from build123d import *

# Parameters (mm, degrees)
SKETCH1_W          = 73.81875
SKETCH1_H          = 114.3
BASE_FLANGE1_DEPTH = 1.5875
EDGE_FLANGE1_DEPTH = 114.3
SKETCH11_R         = 2.45745
CUT_EXTRUDE1_DEPTH = 155.799566224
SKETCH12_R         = 2.45745
CUT_EXTRUDE2_DEPTH = 156.949151494
FILLET1_R          = 2.54


# Sheet-metal steps are written as plain solids
with BuildPart() as part:
    # Sketch1 → Base-Flange1 (new body)
    with BuildSketch(Plane.XY):
        with Locations((36.909375, 57.15)):
            Rectangle(SKETCH1_W, SKETCH1_H)
    extrude(amount=-BASE_FLANGE1_DEPTH)

    # Edge-Flange1 section (across the edge) → Edge-Flange1 (add)
    with BuildSketch(Plane(origin=(-0.79375, 0, -1.5875), x_dir=(1, 0, 0), z_dir=(0, 1, 0))):
        with BuildLine():
            Line((-1.5875, 0.79375), (-1.5875, 72.23125))
            Line((-1.5875, 72.23125), (0, 72.23125))
            Line((0, 72.23125), (0, 0.79375))
            ThreePointArc((0, 0.79375), (0.232483992, 0.232483992), (0.79375, 0))
            Line((0.79375, 0), (0.79375, -1.5875))
            ThreePointArc((0.79375, -1.5875), (-0.890048023, -0.890048023), (-1.5875, 0.79375))
        make_face()
    extrude(amount=EDGE_FLANGE1_DEPTH)

    # Sketch11 → Cut-Extrude1 (cut, through all)
    with BuildSketch(Plane.XY):
        with Locations((30.48, 12.7)):
            Circle(SKETCH11_R)
        with Locations((30.48, 33.02)):
            Circle(SKETCH11_R)
        with Locations((30.48, 53.34)):
            Circle(SKETCH11_R)
        with Locations((30.48, 73.66)):
            Circle(SKETCH11_R)
        with Locations((30.48, 93.98)):
            Circle(SKETCH11_R)
        with Locations((61.11875, 101.6)):
            Circle(SKETCH11_R)
        with Locations((61.11875, 81.28)):
            Circle(SKETCH11_R)
        with Locations((61.11875, 60.96)):
            Circle(SKETCH11_R)
        with Locations((61.11875, 40.64)):
            Circle(SKETCH11_R)
        with Locations((61.11875, 20.32)):
            Circle(SKETCH11_R)
        with BuildLine():
            Line((46.67885, 88.10625), (43.50385, 88.10625))
            ThreePointArc((43.50385, 88.10625), (36.3601, 95.25), (43.50385, 102.39375))
            Line((43.50385, 102.39375), (46.67885, 102.39375))
            ThreePointArc((46.67885, 102.39375), (53.8226, 95.25), (46.67885, 88.10625))
        make_face()
        with BuildLine():
            Line((46.67885, 11.90625), (43.50385, 11.90625))
            ThreePointArc((43.50385, 11.90625), (36.3601, 19.05), (43.50385, 26.19375))
            Line((43.50385, 26.19375), (46.67885, 26.19375))
            ThreePointArc((46.67885, 26.19375), (53.8226, 19.05), (46.67885, 11.90625))
        make_face()
        with BuildLine():
            Line((43.383061388, 65.139055024), (40.208061388, 63.488055024))
            ThreePointArc((40.208061388, 63.488055024), (36.3601, 57.15), (40.208061388, 50.811944976))
            Line((40.208061388, 50.811944976), (43.383061388, 49.160944976))
            ThreePointArc((43.383061388, 49.160944976), (50.386199064, 49.392550378), (53.8226, 55.499))
            Line((53.8226, 55.499), (53.8226, 58.801))
            ThreePointArc((53.8226, 58.801), (50.386199064, 64.907449622), (43.383061388, 65.139055024))
        make_face()
    extrude(amount=-CUT_EXTRUDE1_DEPTH, mode=Mode.SUBTRACT)

    # Sketch12 → Cut-Extrude2 (cut, through all)
    with BuildSketch(Plane.ZY.offset(2.38125)):
        with Locations((-61.11875, 12.7)):
            Circle(SKETCH12_R)
        with Locations((-61.11875, 33.02)):
            Circle(SKETCH12_R)
        with Locations((-61.11875, 53.34)):
            Circle(SKETCH12_R)
        with Locations((-61.11875, 73.66)):
            Circle(SKETCH12_R)
        with Locations((-61.11875, 93.98)):
            Circle(SKETCH12_R)
        with Locations((-32.86125, 73.66)):
            Circle(SKETCH12_R)
        with Locations((-32.86125, 40.64)):
            Circle(SKETCH12_R)
        with Locations((-24.2951, 95.25)):
            Circle(SKETCH12_R)
        with Locations((-24.2951, 19.05)):
            Circle(SKETCH12_R)
        with BuildLine():
            Line((-35.56635, 58.801), (-35.56635, 55.499))
            ThreePointArc((-35.56635, 55.499), (-42.7101, 48.35525), (-49.85385, 55.499))
            Line((-49.85385, 55.499), (-49.85385, 58.801))
            ThreePointArc((-49.85385, 58.801), (-42.7101, 65.94475), (-35.56635, 58.801))
        make_face()
        with BuildLine():
            Line((-42.7101, 102.39375), (-39.5351, 102.39375))
            ThreePointArc((-39.5351, 102.39375), (-32.39135, 95.25), (-39.5351, 88.10625))
            Line((-39.5351, 88.10625), (-42.7101, 88.10625))
            ThreePointArc((-42.7101, 88.10625), (-49.85385, 95.25), (-42.7101, 102.39375))
        make_face()
        with BuildLine():
            Line((-42.7101, 26.19375), (-39.5351, 26.19375))
            ThreePointArc((-39.5351, 26.19375), (-32.39135, 19.05), (-39.5351, 11.90625))
            Line((-39.5351, 11.90625), (-42.7101, 11.90625))
            ThreePointArc((-42.7101, 11.90625), (-49.85385, 19.05), (-42.7101, 26.19375))
        make_face()
    extrude(amount=-CUT_EXTRUDE2_DEPTH, mode=Mode.SUBTRACT)

    # Fillet1
    fillet1_edges = [part.edges().sort_by_distance(p)[0] for p in [
        (-1.5875, 0, -73.81875),
        (-1.5875, 114.3, -73.81875),
        (73.81875, 114.3, -0.79375),
        (73.81875, 0, -0.79375),
    ]]
    fillet(fillet1_edges, radius=FILLET1_R)


solid = part.part
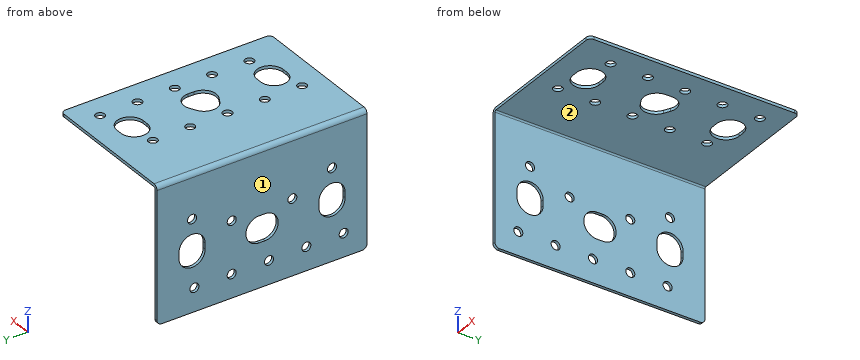
Verification items for the finished model (mm, model axes). Face numbers are marked on the shaded views. A direction names the side the tool comes from. Give positions to 0.01 mm unless a question says otherwise; leave off trailing zeros. Loops run counter-clockwise (first coordinate to the right, second up) from the corner with the lowest first, then second, coordinate; pieces in that order, holes last.
1) Sectioned sample at B-B, the plane x = 48. Enter the section's corners in (y, z), then the cut area to 3 significant figures.
2) Depth check by flat-ended pin: pin 1 Ø10 at (x, y) = (36, 39.5) entering from +Z; pin 2 Ø3 at (y, z) = (81, -59.5) entering from +X; pin 3 Ø0.8 at (y, z) = (56.5, -0.5) entering from -X; pin 4 Ø6 at (x, y) = (64.5, 42) entering from -Z. Enter the tip coordinate at first touch or a pass-through.
3) Set-up check for the marked faces 1 and 2: record each of +Z, -Z, +X, -X, +Y, -Y from which the full face is reachable in a straight line by a thin tool's end or side.
4) Sectioned sample at C-C, the plane y = 86.5. Enter the section's corners in (x, z).
5) Thickness scan on line 1 along Y through (x, z) = (30.48, -0.6); line 2 along X through (y, z) = (34, -50); line 3 along Z through (x, y) = (21, 42.5). Record the ranges inside material, lowest first.
6) Sectioned sample at D-D, the plane y = 53.34. Enter the section's corners in (x, z).
7) Sectioned sample at A-A, the plane y = 73.66. Enter the section's corners in (x, z), then the cut area to 3 significant figures.
Answers:
1. outline: (0, -1.59) - (12.03, -1.59) - (12.03, 0) - (0, 0) - close; (26.07, -1.59) - (48.48, -1.59) - (48.48, 0) - (26.07, 0) - close; (65.82, -1.59) - (88.23, -1.59) - (88.23, 0) - (65.82, 0) - close; (102.27, -1.59) - (114.3, -1.59) - (114.3, 0) - (102.27, 0) - close
1. area: 109 mm2
2. pin 1: stops at z = 0
2. pin 2: stops at x = -0.79
2. pin 3: stops at x = -1.86
2. pin 4: stops at z = -1.59
3. face 1: +Z, -Z, -X, +Y, -Y
3. face 2: -Z, +X, +Y, -Y
4. outline: (-2.38, -73.82) - (-0.79, -73.82) - (-0.79, -2.38) arc R0.79 cw to (0, -1.59) - (73.82, -1.59) - (73.82, 0) - (0, 0) arc R2.38 ccw to (-2.38, -2.38) - close
5. line 1: y = 0 to 10.24, 15.16 to 30.56, 35.48 to 50.88, 55.8 to 71.2, 76.12 to 91.52, 96.44 to 114.3
5. line 2: x = -2.38 to -0.79
5. line 3: z = -1.59 to 0
6. outline: (-2.38, -73.82) - (-0.79, -73.82) - (-0.79, -63.58) - (-2.38, -63.58) - close; (-2.38, -58.66) - (-0.79, -58.66) - (-0.79, -49.52) - (-2.38, -49.52) - close; (-2.38, -35.9) - (-0.79, -35.9) - (-0.79, -2.38) arc R0.79 cw to (0, -1.59) - (28.02, -1.59) - (28.02, 0) - (0, 0) arc R2.38 ccw to (-2.38, -2.38) - close; (32.94, -1.59) - (37.46, -1.59) - (37.46, 0) - (32.94, 0) - close; (53.49, -1.59) - (73.82, -1.59) - (73.82, 0) - (53.49, 0) - close
7. outline: (-2.38, -73.82) - (-0.79, -73.82) - (-0.79, -63.58) - (-2.38, -63.58) - close; (-2.38, -58.66) - (-0.79, -58.66) - (-0.79, -35.32) - (-2.38, -35.32) - close; (-2.38, -30.4) - (-0.79, -30.4) - (-0.79, -2.38) arc R0.79 cw to (0, -1.59) - (28.02, -1.59) - (28.02, 0) - (0, 0) arc R2.38 ccw to (-2.38, -2.38) - close; (32.94, -1.59) - (73.82, -1.59) - (73.82, 0) - (32.94, 0) - close
7. area: 211 mm2
